Here's how the part is built. I have some questions about the finished solid (model axes, mm). A direction names the side the tool comes from. Coordinates: 2 decimals unless noted, no trailing zeros. Loops run counter-clockwise (first coordinate to the right, second up) from the corner with the lowest first, then second, coordinate; pieces in that order, holes last. Notation, with made-up numbers: M 24.5,23 L 59.5,23 A28 ccw 59.5,54 Z; hole C 89.5,21 d8. An arc over 180 degrees is marked long. Use CSV: the item, a comma, the result in double quotes. Start each with the question number.
Q1. If we section it at A-A (y = 40): Please give me the cut outline in (x, z) (3 decimals), and give its area (3 significant figures).
Q2. If we section it at C-C (x = -46.5): Please give me the cut outline in (y, z) (3 decimals).
Q3. If we section it at B-B (y = 0): Please give me the cut outline in (x, z) (3 decimals).
Q4. Which directions (+Z, -Z, +X, -X, +Y, -Y) give clear straight access to the entire face, cutting with the end or side of a thin tool? Please do faces 1 (the flat face through (-62, 10, 38.1)), 2 (the cylindrical face through (-70.97, 33.1, 19.11)), 3 (the flat face through (-50.8, 3, 8)), 4 (the flat face through (-70, 30.795, 18)).
Q5. If we mould it in two halves opening along Z, with no side actions, what happens to faces 5 (the cylindrical face through (-70.97, 35.79, 29)), 6 (the flat face through (-64, -24.13, 23)), 7 (the flat face through (-19, 32, 25.4)), 8 (the flat face through (-50, 19, 0))? For each: +Z half, -Z half, draft (parallel to the pull), parting line (faces both ways), or undercut.
Q6. Please list where these lines run through material, in increasing order: probe 1 along Y at (x, z) = (-75.25, 25.4) (3 decimals); probe 2 along Z at (x, y) = (-71, 30.5); probe 3 along Y at (x, z) = (-56.5, 21) (3 decimals). Write a range as [from, to].
Q7. If we section it at D-D (y = 26): Please give me the cut outline in (x, z) (3 decimals), and give its area (3 significant figures).
Q8. For pin 1 Ø10 at (x, z) = (-7, 5) entering from -Y (3 decimals); pin 2 Ø2 at (y, z) = (20, 34.5) entering from +X; pin 3 Ø4 at (y, z) = (36.5, 32) entering from +X, each with a flat end and sliding along its axis, tell me the tip position at first contact or that it passes through.
from build123d import *

# Parameters (mm, degrees)
SKETCH1_R                       = 19.05
SKETCH1_W                       = 152.4
SKETCH1_H                       = 38.1
BOSS_EXTRUDE1_DEPTH             = 25.4
SKETCH4_W                       = 25.4
SKETCH4_H                       = 69.85
BOSS_EXTRUDE3_DEPTH             = 19.05
BOSS_EXTRUDE3_DIRECTION_2_REACH = 102.402
SKETCH5_R                       = 6.985
SKETCH5_R_2                     = 1.905
CUT_EXTRUDE1_DEPTH              = 25.4
SKETCH13_W                      = 63.5
SKETCH13_H                      = 69.85
BOSS_EXTRUDE6_DEPTH             = 25.4
SKETCH7_W                       = 50.8
SKETCH7_H                       = 55.88
CUT_EXTRUDE2_DEPTH              = 25.4
SKETCH8_W                       = 25.4
SKETCH8_H                       = 39.99992
CUT_EXTRUDE3_DEPTH              = 23.400004
SKETCH9_W                       = 25.4
SKETCH9_H                       = 7.94004
CUT_EXTRUDE4_DEPTH              = 14.800072
SKETCH10_W                      = 2.54
SKETCH10_H                      = 7.94004
CUT_EXTRUDE5_DEPTH              = 8.599932
SKETCH11_R                      = 3.175
CUT_EXTRUDE6_DEPTH              = 109.664809851
BOSS_EXTRUDE7_DEPTH             = 55.88
CUT_EXTRUDE7_DEPTH              = 127.203753906
SKETCH16_W                      = 57.15
SKETCH16_H                      = 34.925
CUT_EXTRUDE8_DEPTH              = 93.422499425
SKETCH17_R                      = 3.175
CUT_EXTRUDE9_DEPTH              = 95.878860264


with BuildPart() as part:
    # Sketch1 → Boss-Extrude1 (new body)
    with BuildSketch(Plane.XY):
        with Locations((76.2, 0)):
            Circle(SKETCH1_R)
        Rectangle(SKETCH1_W, SKETCH1_H)
    extrude(amount=BOSS_EXTRUDE1_DEPTH)

    # Sketch4 → Boss-Extrude3 (add)
    with BuildSketch(Plane.XY.offset(25.4)):
        with Locations((-63.5, 10.795)):
            Rectangle(SKETCH4_W, SKETCH4_H)
    extrude(amount=BOSS_EXTRUDE3_DEPTH)

    # Boss-Extrude3 direction 2: up to this face of the body (flat: up to its plane)
    boss_extrude3_direction_2_end = Plane(part.part.faces().sort_by_distance((7.534927708, 0, 0))[0])
    # Sketch4 → Boss-Extrude3 direction 2 (add, up to the picked face)
    with BuildSketch(Plane.XY.offset(25.4), mode=Mode.PRIVATE) as boss_extrude3_direction_2_sk1:
        with Locations((-63.5, 10.795)):
            Rectangle(SKETCH4_W, SKETCH4_H)
    boss_extrude3_direction_2_tool1 = split(extrude(boss_extrude3_direction_2_sk1.sketch, amount=-BOSS_EXTRUDE3_DIRECTION_2_REACH, mode=Mode.PRIVATE), bisect_by=boss_extrude3_direction_2_end, keep=Keep.BOTH, mode=Mode.PRIVATE)
    add(boss_extrude3_direction_2_tool1.solids().sort_by(Axis((-63.5, 10.795, 25.4), (0, 0, -1)))[0])

    # Sketch5 → Cut-Extrude1 (cut)
    with BuildSketch(Plane.ZY.offset(76.2)):
        with Locations((25.4, 0)):
            Circle(SKETCH5_R)
        with Locations((30.39999, -14.500098)):
            Circle(SKETCH5_R_2)
        with Locations((30.39999, 34.499804)):
            Circle(SKETCH5_R_2)
        with Locations(Location((20.40001, 34.499804, 0), (0, 0, 90))):
            Circle(SKETCH5_R_2)
        with Locations(Location((20.40001, -14.500098, 0), (0, 0, 90))):
            Circle(SKETCH5_R_2)
    extrude(amount=-CUT_EXTRUDE1_DEPTH, mode=Mode.SUBTRACT)

    # Sketch13 → Boss-Extrude6 (add)
    with BuildSketch(Plane.XY.offset(25.4)):
        with Locations((-19.05, 10.795)):
            Rectangle(SKETCH13_W, SKETCH13_H)
    extrude(amount=-BOSS_EXTRUDE6_DEPTH)

    # Sketch7 → Cut-Extrude2 (cut)
    with BuildSketch(Plane.XY.offset(25.4)):
        with Locations((-25.4, 10.795)):
            Rectangle(SKETCH7_W, SKETCH7_H)
    extrude(amount=-CUT_EXTRUDE2_DEPTH, mode=Mode.SUBTRACT)

    # Sketch8 → Cut-Extrude3 (cut)
    with BuildSketch(Plane(origin=(-50.8, 0, 0), x_dir=(0, 0, -1), z_dir=(1, 0, 0))):
        with Locations((-25.4, 10.795)):
            Rectangle(SKETCH8_W, SKETCH8_H)
    extrude(amount=-CUT_EXTRUDE3_DEPTH, mode=Mode.SUBTRACT)

    # Sketch9 → Cut-Extrude4 (cut)
    with BuildSketch(Plane(origin=(-50.8, 0, 0), x_dir=(0, 0, -1), z_dir=(1, 0, 0))):
        with Locations((-25.4, 34.76498)):
            Rectangle(SKETCH9_W, SKETCH9_H)
        with Locations((-25.4, -13.17498)):
            Rectangle(SKETCH9_W, SKETCH9_H)
    extrude(amount=-CUT_EXTRUDE4_DEPTH, mode=Mode.SUBTRACT)

    # Sketch10 → Cut-Extrude5 (cut)
    with BuildSketch(Plane(origin=(-65.600072, 0, 0), x_dir=(0, 0, -1), z_dir=(1, 0, 0))):
        with Locations((-25.4, -13.17498)):
            Rectangle(SKETCH10_W, SKETCH10_H)
        with Locations((-25.4, 34.76498)):
            Rectangle(SKETCH10_W, SKETCH10_H)
    extrude(amount=-CUT_EXTRUDE5_DEPTH, mode=Mode.SUBTRACT)

    # Sketch11 → Cut-Extrude6 (cut, through all)
    with BuildSketch(Plane.XY.offset(25.4)):
        with Locations((76.2, 0)):
            Circle(SKETCH11_R)
    extrude(amount=-CUT_EXTRUDE6_DEPTH, mode=Mode.SUBTRACT)

    # Sketch14 → Boss-Extrude7 (add)
    with BuildSketch(Plane(origin=(0, -17.145, 0), x_dir=(1, 0, 0), z_dir=(0, 1, 0))):
        Polygon((-50.8, -12.7), (-25.4, -12.7), (-25.4, -25.4), (0, -25.4), (0, 0), (-50.8, 0), align=None)
    extrude(amount=BOSS_EXTRUDE7_DEPTH)

    # Sketch15 → Cut-Extrude7 (cut, through all)
    with BuildSketch(Plane(origin=(0, 45.72, 0), x_dir=(1, 0, 0), z_dir=(0, 1, 0))):
        with BuildLine():
            Line((-6.35, 0), (95.25, 0))
            Line((95.25, 0), (95.25, -25.4))
            Line((95.25, -25.4), (-6.35, -25.4))
            ThreePointArc((-6.35, -25.4), (6.35, -12.7), (-6.35, 0))
        make_face()
    extrude(amount=-CUT_EXTRUDE7_DEPTH, mode=Mode.SUBTRACT)

    # Sketch16 → Cut-Extrude8 (cut, through all)
    with BuildSketch(Plane.XY.offset(25.4)):
        with Locations((-22.225, -6.6675)):
            Rectangle(SKETCH16_W, SKETCH16_H)
    extrude(amount=-CUT_EXTRUDE8_DEPTH, mode=Mode.SUBTRACT)

    # Sketch17 → Cut-Extrude9 (cut, through all)
    with BuildSketch(Plane.XZ.offset(-10.795)):
        with Locations(Location((-6.35, 12.7, 0), (0, 0, 270))):
            Circle(SKETCH17_R)
    extrude(amount=-CUT_EXTRUDE9_DEPTH, mode=Mode.SUBTRACT)


solid = part.part
Results below:
1,outline,"M -76.2,0 L -6.35,0 A12.7 ccw -6.35,25.4 L -50.8,25.4 L -50.8,44.45 L -76.2,44.45 Z; hole C -6.35,12.7 d6.35"
1,area,"2,480 mm^2"
2,outline,"M 10.795,0 L 45.72,0 L 45.72,25.4 L 38.735,25.4 L 38.735,12.7 L 10.795,12.7 Z"
3,outline,"M -76.2,0 L -50.8,0 L -50.8,12.7 L -74.2,12.7 L -74.2,18.415 L -76.2,18.415 Z; M -76.2,32.385 L -74.2,32.385 L -74.2,38.1 L -50.8,38.1 L -50.8,44.45 L -76.2,44.45 Z"
4,face 1,"+X"
4,face 2,"-X"
4,face 3,"+Z, +X, -Y"
4,face 4,"none"
5,face 5,"undercut"
5,face 6,"draft"
5,face 7,"+Z half"
5,face 8,"-Z half"
6,probe 1,"[-24.13, -6.985], [6.985, 45.72]"
6,probe 2,"[0, 12.7], [38.1, 44.45]"
6,probe 3,"[-24.13, -17.145], [38.735, 45.72]"
7,outline,"M -76.2,0 L -6.35,0 A12.7 ccw -6.35,25.4 L -25.4,25.4 L -25.4,12.7 L -74.2,12.7 L -74.2,38.1 L -50.8,38.1 L -50.8,44.45 L -76.2,44.45 Z; hole C -6.35,12.7 d6.35"
7,area,"1,560 mm^2"
8,pin 1,"y = 10.795"
8,pin 2,"x = -74.2"
8,pin 3,"x = -65.6"
